from build123d import *

# Parameters (mm, degrees)
SKETCH1_R                  = 28.3
BOSS_EXTRUDE1_DEPTH        = 5
SKETCH4_R                  = 11.5
BOSS_EXTRUDE2_DEPTH        = 30
SKETCH10_R                 = 7.95
CUT_EXTRUDE4_DEPTH         = 36
F_4_40_TAPPED_HOLE2_REACH  = 42.359
F_4_40_TAPPED_HOLE2_BORE_R = 1.1303
CIRPATTERN3_COUNT          = 3


with BuildPart() as part:
    # Sketch1 → Boss-Extrude1 (new body)
    with BuildSketch(Plane.XY):
        Circle(SKETCH1_R)
    extrude(amount=BOSS_EXTRUDE1_DEPTH)

    # Sketch4 → Boss-Extrude2 (add)
    with BuildSketch(Plane(origin=(0, 0, 0), x_dir=(-1, 0, 0), z_dir=(0, 0, -1))):
        with Locations(Location((0, 0, 0), (0, 0, 180))):  # turned: the seam where the file's is
            Circle(SKETCH4_R)
    extrude(amount=BOSS_EXTRUDE2_DEPTH)

    # Sketch10 → Cut-Extrude4 (cut, through all)
    with BuildSketch(Plane(origin=(0, 0, -30), x_dir=(-1, 0, 0), z_dir=(0, 0, -1))):
        Circle(SKETCH10_R)
    extrude(amount=-CUT_EXTRUDE4_DEPTH, mode=Mode.SUBTRACT)

    # #4-40 Tapped Hole2 bore (on position points) → #4-40 Tapped Hole2 (cut, up to next)
    with BuildSketch(Plane(origin=(-11.49770937, 0.22951958, -23.090859569), x_dir=(-0.019958224, -0.999800815, 0), z_dir=(-0.999800815, 0.019958224, 0)), mode=Mode.PRIVATE) as f_4_40_tapped_hole2_sk1:
        Circle(F_4_40_TAPPED_HOLE2_BORE_R)
    f_4_40_tapped_hole2_tool1 = extrude(f_4_40_tapped_hole2_sk1.sketch, amount=-F_4_40_TAPPED_HOLE2_REACH, mode=Mode.PRIVATE) & part.part
    f_4_40_tapped_hole2 = f_4_40_tapped_hole2_tool1.solids().sort_by_distance((-11.497709, 0.22952, -23.09086))[0]
    add(f_4_40_tapped_hole2, mode=Mode.SUBTRACT)

    # CirPattern3: #4-40 Tapped Hole2 ×3 about axis
    cirpattern3_axis = Axis((0, 0, -30), (0, 0, 1))
    for i in range(1, CIRPATTERN3_COUNT):
        add(f_4_40_tapped_hole2.rotate(cirpattern3_axis, i * 360 / CIRPATTERN3_COUNT), mode=Mode.SUBTRACT)


solid = part.part
The model under review builds one solid part; all positions refer to its coordinate system, in mm. A direction names the side the tool comes from. Round coordinates to 2 decimals unless told otherwise and drop trailing zeros. Order: outer loops, then holes, each group sorted by start corner. A loop starts at its lowest first (then second) coordinate and runs counter-clockwise, first axis right, second up. Notation, with made-up numbers: (46.25, -31.5) -> (81.25, -31.5) arc R18 cw to (81.25, -18.5) -> close; hole circle Ø9 at (7.5, -5). An arc over 180 degrees is marked (long way). Write item = value, one per line. Start each with the question number.
Item 1: Mouldability with a two-part tool opening along X and no side actions: class faces 1 (the face through (6, -6, 5)), 2 (the face through (13.059, -25.107, 2.465)), 3 (the face through (5.143, -8.253, -24.094)) as released by +X, released by -X, zero draft, split by the parting line, or undercut.
Item 2: Clearance check with flat-ended pins moving along their axes: pin 1 Ø5 at (x, z) = (8.5, -10) entering from -Y; pin 2 Ø12 at (x, y) = (-16.5, 18.5) entering from -Z; pin 3 Ø4 at (y, z) = (4, -16.5) entering from +X. State where each tip first meets the part, or that it passes through.
Item 3: For faces 4 (the face through (1.72, -7.76, -12.74)), 5 (the face through (0, -12, 0)), list the 3-axis set-ups (+Z, -Z, +X, -X, +Y, -Y) from which the entire face can be reached by the end or side of a thin tool; tool diameter is ignored.
Item 4: For line 1 along Y through (x, z) = (0, -20); line 2 along Z through (x, y) = (-17, 12.5); line 3 along X through (y, z) = (-2, -6), list the stretches that pass through material, from the lowest coordinate up.
Item 5: Consider section B-B on z = -3. Write out the cut boundary in (x, y).
Item 6: Consider section C-C on y = 0. Count the separate pieces of the cut face and the enclosed holes in it, plus the area to 3 significant figures.
Item 7: Consider section D-D on y = -15.5. Write out the cut boundary in (x, z), plus the area to 3 significant figures.
Item 8: Consider section A-A on x = 0. Write out the cut boundary in (y, z), plus the area to 4 significant figures.
Conclusion:
q1.face_1 = zero draft
q1.face_2 = split by the parting line
q1.face_3 = undercut
q2.pin_1 = -9.81
q2.pin_2 = 0
q2.pin_3 = 11.32
q3.face_4 = +Z, -Z
q3.face_5 = -Z
q4.line_1 = -11.5 to -7.95, 7.95 to 11.5
q4.line_2 = 0 to 5
q4.line_3 = -11.32 to -7.69, 7.69 to 11.32
q5.outline = circle Ø23 at (0, 0); hole circle Ø15.9 at (0, 0)
q6.separate_pieces = 3
q6.enclosed_holes = 0
q6.area = 409 mm2
q7.outline = (-23.68, 0) -> (23.68, 0) -> (23.68, 5) -> (-23.68, 5) -> close
q7.area = 237 mm2
q8.outline = (-28.3, 0) -> (-11.5, 0) -> (-11.5, -30) -> (-7.95, -30) -> (-7.95, 5) -> (-28.3, 5) -> close; (7.95, -30) -> (11.5, -30) -> (11.5, 0) -> (28.3, 0) -> (28.3, 5) -> (7.95, 5) -> close
q8.area = 416.5 mm2
